The listing builds one solid part. Answer for the finished solid, in the listing's coordinates (mm). A direction names the side the tool comes from. Round coordinates to 2 decimals unless told otherwise and drop trailing zeros. Write each loop counter-clockwise with the first axis right and the second up, starting at its lowest first coordinate (ties: lowest second). Pieces come first, ordered by that corner, then holes. Notation, with made-up numbers: (32.25, 42.25) - (65.25, 42.25) arc R19 cw to (65.25, 68.25) - close; hole circle Ø10 at (-7, -6.75). An arc over 180 degrees is marked (long way). Use a Markdown table: item, result. Add a question column.
1) A cutting plane is placed at B-B (y = 0.7). Give the vertices of the cut face in (x, z), then the cut area to 3 significant figures.
2) A cutting plane is placed at A-A (z = 6.75). Give the vertices of the cut face in (x, y), then the cut area to 3 significant figures.
3) Find the intervals of material crossed by probe 1 along X at (y, z) = (0.25, 10.75); probe 2 along X at (y, z) = (2, 0.5); probe 3 along Z at (x, y) = (-189, 1.25), in increasing order. Write a range as from..to.
4) A cutting plane is placed at C-C (x = -170.5). Give the vertices of the cut face in (y, z).
5) A cutting plane is placed at D-D (z = -8). Give the vertices of the cut face in (x, y).
6) A tool of negligible diameter and unlimited length cuts with its end or side. For faces 5 (the flat face through (-177, 1, 10.402)), 6 (the flat face through (-150, 1, -9.598)), 7 (the flat face through (-139, 1, -3.598)), 8 (the flat face through (-177, 1, -9.598)), from which of +Z, -Z, +X, -X, +Y, -Y can it reach the whole face along a straight path? Write none if from no direction.
7) Determine the mould class of faces 1 (the flat face through (-145.732, 1, 11)), 2 (the flat face through (-142, 1, 12.402)), 3 (the flat face through (-139.732, 1, 0)), 4 (the flat face through (-153.732, 1, 11)) for opening direction X: +X half, -X half, draft (parallel to the pull), parting line (faces both ways), or undercut.
8) Each of these flat-tipped pins is pushed along its axis until it touches: P1, Ø8.5, axis at x = -149.73, z = 0.4, coming from the -Y side; P2, Ø0.6, axis at y = 1, z = -10.5, coming from the -X side; P3, Ø1.1, axis at x = -176.5, y = 1, coming from the +Z side; P4, Ø0.7, axis at y = 1, z = 0, coming from the +X side. Where does it stop, or does it pass through?
```python
from build123d import *

# Parameters (mm, degrees)
SKETCH1_R           = 7
BOSS_EXTRUDE1_DEPTH = 2.2


with BuildPart() as part:
    # Sketch1 → Boss-Extrude1 (new body)
    with BuildSketch(Plane(origin=(0, 0, 0), x_dir=(1, 0, 0), z_dir=(0, 1, 0))):
        Polygon((-137.731808477, 3.597712716), (-137.731808477, 11.597712716), (-145.731808477, 11.597712716), (-145.731808477, 9.597712716), (-153.731808477, 9.597712716), (-153.731808477, 11.597712716), (-161.731808477, 11.597712716), (-161.731808477, 9.597712716), (-191.731808477, 9.597712716), (-196.731808477, 4.597712716), (-196.731808477, -5.402287284), (-191.731808477, -10.402287284), (-161.731808477, -10.402287284), (-161.731808477, -12.402287284), (-153.731808477, -12.402287284), (-153.731808477, -10.402287284), (-145.731808477, -10.402287284), (-145.731808477, -12.402287284), (-137.731808477, -12.402287284), (-137.731808477, -4.402287284), (-139.731808477, -4.402287284), (-139.731808477, 3.597712716), align=None)
        with Locations(Location((-149.731808477, -0.402287284, 0), (0, 0, 270))):
            Circle(SKETCH1_R, mode=Mode.SUBTRACT)
    extrude(amount=BOSS_EXTRUDE1_DEPTH)


solid = part.part
```
Entries:
| question | item | result |
|---|---|---|
| 1 | outline | (-196.73, -4.6) - (-191.73, -9.6) - (-161.73, -9.6) - (-161.73, -11.6) - (-153.73, -11.6) - (-153.73, -9.6) - (-145.73, -9.6) - (-145.73, -11.6) - (-137.73, -11.6) - (-137.73, -3.6) - (-139.73, -3.6) - (-139.73, 4.4) - (-137.73, 4.4) - (-137.73, 12.4) - (-145.73, 12.4) - (-145.73, 10.4) - (-153.73, 10.4) - (-153.73, 12.4) - (-161.73, 12.4) - (-161.73, 10.4) - (-191.73, 10.4) - (-196.73, 5.4) - close; hole circle Ø14 at (-149.73, 0.4) |
| 1 | area | 1,050 mm² |
| 2 | outline | (-195.38, 0) - (-152.68, 0) - (-152.68, 2.2) - (-195.38, 2.2) - close; (-146.78, 0) - (-137.73, 0) - (-137.73, 2.2) - (-146.78, 2.2) - close |
| 2 | area | 114 mm² |
| 3 | probe 1 | x = -161.73..-153.73, -145.73..-137.73 |
| 3 | probe 2 | x = -196.73..-156.73, -142.73..-139.73 |
| 3 | probe 3 | z = -9.6..10.4 |
| 4 | outline | (0, -9.6) - (2.2, -9.6) - (2.2, 10.4) - (0, 10.4) - close |
| 5 | outline | (-193.33, 0) - (-137.73, 0) - (-137.73, 2.2) - (-193.33, 2.2) - close |
| 6 | face 5 | +Z, -X, +Y, -Y |
| 6 | face 6 | -Z, +Y, -Y |
| 6 | face 7 | +X, +Y, -Y |
| 6 | face 8 | -Z, -X, +Y, -Y |
| 7 | face 1 | undercut |
| 7 | face 2 | draft |
| 7 | face 3 | +X half |
| 7 | face 4 | undercut |
| 8 | P1 | passes through |
| 8 | P2 | stops at x = -161.73 |
| 8 | P3 | stops at z = 10.4 |
| 8 | P4 | stops at x = -139.73 |
